from build123d import *

# Parameters (mm, degrees)
CUT_EXTRUDE1_START = 1651
CUT_EXTRUDE1_DEPTH = 177.8
CUT_EXTRUDE2_REACH = 1831.153
SKETCH2_R          = 2.413
CUT_EXTRUDE3_REACH = 1831.153
SKETCH5_R          = 2.413
SKETCH6_R          = 2.413
CUT_EXTRUDE6_DEPTH = 12.7
SKETCH7_R          = 2.413
CUT_EXTRUDE7_DEPTH = 12.7
CUT_EXTRUDE8_REACH = 1831.153
SKETCH8_R          = 2.413
CUT_EXTRUDE9_REACH = 1831.153
SKETCH9_R          = 2.413


with BuildPart() as part:
    # Cut-Extrude1: read off the stored shape, not the designer's step
    # Cut-Extrude1 outline → Cut-Extrude1 (new body)
    with BuildSketch(Plane.XY.offset(CUT_EXTRUDE1_START)):
        with BuildLine():
            Line((0, 25.146), (0, 0.254))
            ThreePointArc((0, 0.254), (0.074394878, 0.074394878), (0.254, 0))
            Line((0.254, 0), (25.146, 0))
            ThreePointArc((25.146, 0), (25.325605122, 0.074394878), (25.4, 0.254))
            Line((25.4, 0.254), (25.4, 25.146))
            ThreePointArc((25.4, 25.146), (25.325605122, 25.325605122), (25.146, 25.4))
            Line((25.146, 25.4), (0.254, 25.4))
            ThreePointArc((0.254, 25.4), (0.074394878, 25.325605122), (0, 25.146))
        make_face()
        with BuildLine():
            ThreePointArc((4.7625, 3.175), (3.639967985, 3.639967985), (3.175, 4.7625))
            Line((3.175, 4.7625), (3.175, 20.6375))
            ThreePointArc((3.175, 20.6375), (3.639967985, 21.760032015), (4.7625, 22.225))
            Line((4.7625, 22.225), (20.6375, 22.225))
            ThreePointArc((20.6375, 22.225), (21.760032015, 21.760032015), (22.225, 20.6375))
            Line((22.225, 20.6375), (22.225, 4.7625))
            ThreePointArc((22.225, 4.7625), (21.760032015, 3.639967985), (20.6375, 3.175))
            Line((20.6375, 3.175), (4.7625, 3.175))
        make_face(mode=Mode.SUBTRACT)
    extrude(amount=CUT_EXTRUDE1_DEPTH)

    # Sketch2 → Cut-Extrude2 (cut, up to next)
    with BuildSketch(Plane(origin=(25.4, 0, 0), x_dir=(0, 0, -1), z_dir=(1, 0, 0)), mode=Mode.PRIVATE) as cut_extrude2_sk1:
        with Locations((-1665.216211664, 12.7)):
            Circle(SKETCH2_R)
    cut_extrude2_tool1 = extrude(cut_extrude2_sk1.sketch, amount=-CUT_EXTRUDE2_REACH, mode=Mode.PRIVATE) & part.part
    # Sketch2 → Cut-Extrude2 (cut, up to next)
    with BuildSketch(Plane(origin=(25.4, 0, 0), x_dir=(0, 0, -1), z_dir=(1, 0, 0)), mode=Mode.PRIVATE) as cut_extrude2_sk2:
        with Locations((-1684.266211664, 12.7)):
            Circle(SKETCH2_R)
    cut_extrude2_tool2 = extrude(cut_extrude2_sk2.sketch, amount=-CUT_EXTRUDE2_REACH, mode=Mode.PRIVATE) & part.part
    add(cut_extrude2_tool1.solids().sort_by_distance((25.4, 12.7, 1665.216212))[0], mode=Mode.SUBTRACT)
    add(cut_extrude2_tool2.solids().sort_by_distance((25.4, 12.7, 1684.266212))[0], mode=Mode.SUBTRACT)

    # Sketch5 → Cut-Extrude3 (cut, up to next)
    with BuildSketch(Plane.XZ, mode=Mode.PRIVATE) as cut_extrude3_sk1:
        with Locations(Location((12.7, 1684.02, 0), (0, 0, 90))):
            Circle(SKETCH5_R)
    cut_extrude3_tool1 = extrude(cut_extrude3_sk1.sketch, amount=-CUT_EXTRUDE3_REACH, mode=Mode.PRIVATE) & part.part
    # Sketch5 → Cut-Extrude3 (cut, up to next)
    with BuildSketch(Plane.XZ, mode=Mode.PRIVATE) as cut_extrude3_sk2:
        with Locations(Location((12.7, 1664.97, 0), (0, 0, 90))):
            Circle(SKETCH5_R)
    cut_extrude3_tool2 = extrude(cut_extrude3_sk2.sketch, amount=-CUT_EXTRUDE3_REACH, mode=Mode.PRIVATE) & part.part
    add(cut_extrude3_tool1.solids().sort_by_distance((12.7, 0, 1684.02))[0], mode=Mode.SUBTRACT)
    add(cut_extrude3_tool2.solids().sort_by_distance((12.7, 0, 1664.97))[0], mode=Mode.SUBTRACT)

    # Sketch6 → Cut-Extrude6 (cut)
    with BuildSketch(Plane(origin=(0, 25.4, 0), x_dir=(1, 0, 0), z_dir=(0, 1, 0))):
        with Locations((12.7, -1638.3)):
            Circle(SKETCH6_R)
        with Locations(Location((12.7, -1714.5, 0), (0, 0, 270))):
            Circle(SKETCH6_R)
        with Locations(Location((12.7, -1790.7, 0), (0, 0, 270))):
            Circle(SKETCH6_R)
    extrude(amount=-CUT_EXTRUDE6_DEPTH, mode=Mode.SUBTRACT)

    # Sketch7 → Cut-Extrude7 (cut)
    with BuildSketch(Plane.ZY):
        with Locations((1638.3, 12.7)):
            Circle(SKETCH7_R)
        with Locations((1714.5, 12.7)):
            Circle(SKETCH7_R)
        with Locations((1790.7, 12.7)):
            Circle(SKETCH7_R)
    extrude(amount=-CUT_EXTRUDE7_DEPTH, mode=Mode.SUBTRACT)

    # Sketch8 → Cut-Extrude8 (cut, up to next)
    with BuildSketch(Plane(origin=(25.4, 0, 0), x_dir=(0, 0, -1), z_dir=(1, 0, 0)), mode=Mode.PRIVATE) as cut_extrude8_sk1:
        with Locations(Location((-1790.7, 12.7, 0), (0, 0, 180))):
            Circle(SKETCH8_R)
    cut_extrude8_tool1 = extrude(cut_extrude8_sk1.sketch, amount=-CUT_EXTRUDE8_REACH, mode=Mode.PRIVATE) & part.part
    # Sketch8 → Cut-Extrude8 (cut, up to next)
    with BuildSketch(Plane(origin=(25.4, 0, 0), x_dir=(0, 0, -1), z_dir=(1, 0, 0)), mode=Mode.PRIVATE) as cut_extrude8_sk2:
        with Locations((-1803.4, 12.7)):
            Circle(SKETCH8_R)
    cut_extrude8_tool2 = extrude(cut_extrude8_sk2.sketch, amount=-CUT_EXTRUDE8_REACH, mode=Mode.PRIVATE) & part.part
    # Sketch8 → Cut-Extrude8 (cut, up to next)
    with BuildSketch(Plane(origin=(25.4, 0, 0), x_dir=(0, 0, -1), z_dir=(1, 0, 0)), mode=Mode.PRIVATE) as cut_extrude8_sk3:
        with Locations((-1816.1, 12.7)):
            Circle(SKETCH8_R)
    cut_extrude8_tool3 = extrude(cut_extrude8_sk3.sketch, amount=-CUT_EXTRUDE8_REACH, mode=Mode.PRIVATE) & part.part
    add(cut_extrude8_tool1.solids().sort_by_distance((25.4, 12.7, 1790.7))[0], mode=Mode.SUBTRACT)
    add(cut_extrude8_tool2.solids().sort_by_distance((25.4, 12.7, 1803.4))[0], mode=Mode.SUBTRACT)
    add(cut_extrude8_tool3.solids().sort_by_distance((25.4, 12.7, 1816.1))[0], mode=Mode.SUBTRACT)

    # Sketch9 → Cut-Extrude9 (cut, up to next)
    with BuildSketch(Plane.XZ, mode=Mode.PRIVATE) as cut_extrude9_sk1:
        with Locations(Location((12.7, 1816.1, 0), (0, 0, 270))):
            Circle(SKETCH9_R)
    cut_extrude9_tool1 = extrude(cut_extrude9_sk1.sketch, amount=-CUT_EXTRUDE9_REACH, mode=Mode.PRIVATE) & part.part
    # Sketch9 → Cut-Extrude9 (cut, up to next)
    with BuildSketch(Plane.XZ, mode=Mode.PRIVATE) as cut_extrude9_sk2:
        with Locations(Location((12.7, 1803.4, 0), (0, 0, 270))):
            Circle(SKETCH9_R)
    cut_extrude9_tool2 = extrude(cut_extrude9_sk2.sketch, amount=-CUT_EXTRUDE9_REACH, mode=Mode.PRIVATE) & part.part
    # Sketch9 → Cut-Extrude9 (cut, up to next)
    with BuildSketch(Plane.XZ, mode=Mode.PRIVATE) as cut_extrude9_sk3:
        with Locations(Location((12.7, 1790.7, 0), (0, 0, 90))):
            Circle(SKETCH9_R)
    cut_extrude9_tool3 = extrude(cut_extrude9_sk3.sketch, amount=-CUT_EXTRUDE9_REACH, mode=Mode.PRIVATE) & part.part
    add(cut_extrude9_tool1.solids().sort_by_distance((12.7, 0, 1816.1))[0], mode=Mode.SUBTRACT)
    add(cut_extrude9_tool2.solids().sort_by_distance((12.7, 0, 1803.4))[0], mode=Mode.SUBTRACT)
    add(cut_extrude9_tool3.solids().sort_by_distance((12.7, 0, 1790.7))[0], mode=Mode.SUBTRACT)


solid = part.part
The model under review builds one solid part; all positions refer to its coordinate system, in mm. A direction names the side the tool comes from. Round coordinates to 2 decimals unless told otherwise and drop trailing zeros. Loops run counter-clockwise (first coordinate to the right, second up) from the corner with the lowest first, then second, coordinate; pieces in that order, holes last. Notation, with made-up numbers: M 12.25,-33 L 45.25,-33 A21 cw 45.25,-11 Z; hole C 44,56.25 d3. An arc over 180 degrees is marked long. Answer as CSV lines item,"result". Start each with the question number.
Item 1: Consider section D-D (x = 12.7). State how many separate pieces and enclosed holes the cut face has, then the cut area to 3 significant figures.
Item 2: Wall thickness on line 1 (Y direction, x = 17.5, z = 1717.5) (3 decimals); line 2 (Z direction, x = 13, y = 1.25): over which ranges is each line inside the solid? List them lowest first. Write a range as [from, to].
Item 3: Mouldability with a two-part tool opening along Y and no side actions: class faces 4 (the face through (11.975, 1.565, 1793.002)), 5 (the face through (1.565, 13.425, 1793.002)), 6 (the face through (13, 0, 1739)) as released by +Y, released by -Y, zero draft, split by the parting line, or undercut.
Item 4: Consider section A-A (y = 6.75). Write out the cut boundary in (x, z) (3 decimals).
Item 5: Insertion check: P1, Ø4.5, axis at x = 12.7, z = 1816.1, coming from the -Y side (3 decimals). The pin has a flat end and moves straight along its axis. Give the tip position at first contact, or say it passes through.
Item 6: For faces 1 (the face through (13, 3.175, 1739)), 2 (the face through (11.975, 1.565, 1686.322)), 3 (the face through (23.83, 12.81, 1805.81)), list the 3-axis set-ups (+Z, -Z, +X, -X, +Y, -Y) from which the entire face can be reached by the end or side of a thin tool; tool diameter is ignored.
Answer:
1,separate pieces,"9"
1,enclosed holes,"0"
1,area,"1,020 mm^2"
2,line 1,"y = [0, 3.175], [22.225, 25.4]"
2,line 2,"z = [1651, 1662.58], [1667.36, 1681.63], [1686.41, 1788.31], [1793.09, 1801.01], [1805.79, 1813.71], [1818.49, 1828.8]"
3,face 4,"zero draft"
3,face 5,"undercut"
3,face 6,"released by -Y"
4,outline,"M 0,1651 L 3.175,1651 L 3.175,1828.8 L 0,1828.8 Z; M 22.225,1651 L 25.4,1651 L 25.4,1828.8 L 22.225,1828.8 Z"
5,P1,"stops at y = 22.225"
6,face 1,"+Z, -Z"
6,face 2,"-Y"
6,face 3,"+X"
